```python
from build123d import *

# Parameters (mm, degrees)
EXTRUDE_1_DEPTH                = 500
SKETCH_2_W                     = 500
SKETCH_2_H                     = 30
EXTRUDE_2_DEPTH                = 4.65
CUT_EXTRUDE_1_DEPTH            = 501
CUT_EXTRUDE_2_DEPTH            = 501
SKETCH_5_W                     = 6.7
SKETCH_5_H                     = 0.8
CUT_EXTRUDE_3_DEPTH            = 501
CUT_EXTRUDE_4_DEPTH            = 501
CUT_EXTRUDE_5_DEPTH            = 501
CUT_EXTRUDE_6_DEPTH            = 501
SKETCH_9_W                     = 18.238994336
SKETCH_9_H                     = 8
CUT_EXTRUDE_7_DEPTH            = 501
DRAFT_1_ANGLE                  = 45
DRAFT_2_ANGLE                  = 24.775140569
F_4_2_4_2_DIAMETER_HOLE1_D     = 4.2
F_4_2_4_2_DIAMETER_HOLE1_DEPTH = 500
F_6_0_6_DIAMETER_HOLE1_D       = 6
F_6_0_6_DIAMETER_HOLE1_DEPTH   = 500
CHAMFER_1_SIZE                 = 0.6
CHAMFER_1_SIZE2                = 0.279784595
CHAMFER_2_SIZE                 = 0.6
CHAMFER_3_SIZE                 = 1
CHAMFER_4_SIZE                 = 1.5
FILLET_1_R                     = 3


with BuildPart() as part:
    # 스케치1 → 보스-돌출1 (new body)
    with BuildSketch(Plane(origin=(400, 0, 0), x_dir=(0, 0, -1), z_dir=(1, 0, 0))):
        Polygon((-17.85, 38.2), (-17.85, -0.8), (22.5, -0.8), (22.5, 39.2), (-16.85, 39.2), align=None)
    extrude(amount=-EXTRUDE_1_DEPTH)

    # 스케치2 → 보스-돌출2 (add)
    with BuildSketch(Plane.XY.offset(17.85)):
        with Locations((150, 14.2)):
            Rectangle(SKETCH_2_W, SKETCH_2_H)
    extrude(amount=EXTRUDE_2_DEPTH)

    # 스케치3 → 컷-돌출1 (cut, through all)
    with BuildSketch(Plane.ZY.offset(100)):
        Polygon((22.5, 10.8), (22.5, 15.8), (20.1, 15.8), (20.1, 17.4), (14.9, 17.4), (14.9, 9.2), (20.1, 9.2), (20.1, 10.8), align=None)
    extrude(amount=-CUT_EXTRUDE_1_DEPTH, mode=Mode.SUBTRACT)

    # 스케치4 → 컷-돌출2 (cut, through all)
    with BuildSketch(Plane.ZY.offset(100)):
        Polygon((13.5, -0.8), (18.5, -0.8), (18.5, 1.9), (20.1, 1.9), (20.1, 6.9), (11.9, 6.9), (11.9, 1.9), (13.5, 1.9), align=None)
    extrude(amount=-CUT_EXTRUDE_2_DEPTH, mode=Mode.SUBTRACT)

    # 스케치5 → 컷-돌출3 (cut, through all)
    with BuildSketch(Plane.ZY.offset(100)):
        with Locations((0, -0.4)):
            Rectangle(SKETCH_5_W, SKETCH_5_H)
    extrude(amount=-CUT_EXTRUDE_3_DEPTH, mode=Mode.SUBTRACT)

    # 스케치6 → 컷-돌출4 (cut, through all)
    with BuildSketch(Plane.ZY.offset(100)):
        Polygon((-18.5, -0.8), (-13.5, -0.8), (-13.5, 1.9), (-11.9, 1.9), (-11.9, 6.9), (-20.1, 6.9), (-20.1, 1.9), (-18.5, 1.9), align=None)
    extrude(amount=-CUT_EXTRUDE_4_DEPTH, mode=Mode.SUBTRACT)

    # 스케치7 → 컷-돌출5 (cut, through all)
    with BuildSketch(Plane.ZY.offset(100)):
        Polygon((-22.5, 15.8), (-22.5, 10.8), (-20.1, 10.8), (-20.1, 9.2), (-14.9, 9.2), (-14.9, 17.4), (-20.1, 17.4), (-20.1, 15.8), align=None)
    extrude(amount=-CUT_EXTRUDE_5_DEPTH, mode=Mode.SUBTRACT)

    # 스케치8 → 컷-돌출6 (cut, through all)
    with BuildSketch(Plane.ZY.offset(100)):
        with BuildLine():
            Line((-17.85, 36.705493963), (-17.85, 39.2))
            Line((-17.85, 39.2), (-22.5, 39.2))
            Line((-22.5, 39.2), (-22.5, 29.2))
            Line((-22.5, 29.2), (-17.85, 29.2))
            Line((-17.85, 29.2), (-17.85, 31.694506037))
            ThreePointArc((-17.85, 31.694506037), (-19.2, 34.2), (-17.85, 36.705493963))
        make_face()
    extrude(amount=-CUT_EXTRUDE_6_DEPTH, mode=Mode.SUBTRACT)

    # 스케치9 → 컷-돌출7 (cut, through all)
    with BuildSketch(Plane.ZY.offset(100)):
        with Locations((0, 35.2)):
            Rectangle(SKETCH_9_W, SKETCH_9_H)
    extrude(amount=-CUT_EXTRUDE_7_DEPTH, mode=Mode.SUBTRACT)

    # 구배1
    draft_1_faces = [part.faces().sort_by_distance(p)[0] for p in [
        (150, -0.4, 3.35),
        (150, -0.4, -3.35),
    ]]
    draft(draft_1_faces, Plane(origin=(400, 0, 3.35), x_dir=(0, 0, -1), z_dir=(0, -1, 0)), DRAFT_1_ANGLE)

    # 구배2
    draft_2_faces = [part.faces().sort_by_distance(p)[0] for p in [
        (150, 35.2, 9.119497168),
        (150, 35.2, -9.119497168),
    ]]
    draft(draft_2_faces, Plane(origin=(400, 31.2, -9.119497168), x_dir=(0, 0, 1), z_dir=(0, 1, 0)), DRAFT_2_ANGLE)

    # Ø4.2 (4.2) Diameter Hole1
    with Locations(Plane(origin=(400, 0, 0), x_dir=(0, 0, -1), z_dir=(1, 0, 0))):
        with Locations((-7.5, 5.25), (7.5, 5.25), (0, 26)):
            Hole(F_4_2_4_2_DIAMETER_HOLE1_D / 2, depth=F_4_2_4_2_DIAMETER_HOLE1_DEPTH)

    # Ø6.0 (6) Diameter Hole1
    with Locations(Plane.ZY.offset(100)):
        with Locations((16.290651015, 34.2)):
            Hole(F_6_0_6_DIAMETER_HOLE1_D / 2, depth=F_6_0_6_DIAMETER_HOLE1_DEPTH)

    # 모따기1
    chamfer_1_edges = [part.edges().sort_by_distance(p)[0] for p in [
        (400, 26, -2.1),
        (400, 5.25, -9.6),
        (400, 5.25, 5.4),
    ]]
    chamfer_1_side = [part.faces().sort_by_distance(p)[0] for p in [
        (400, 17.793427641, -0.369480422),
    ]]
    chamfer(chamfer_1_edges, length=CHAMFER_1_SIZE, length2=CHAMFER_1_SIZE2, reference=chamfer_1_side[0])

    # 모따기2
    chamfer_2_edges = [part.edges().sort_by_distance(p)[0] for p in [
        (-100, 26, -2.1),
        (-100, 5.25, -9.6),
        (-100, 5.25, 5.4),
    ]]
    chamfer(chamfer_2_edges, length=CHAMFER_2_SIZE)

    # 모따기3
    chamfer_3_edges = [part.edges().sort_by_distance(p)[0] for p in [
        (150, 39.2, -17.85),
    ]]
    chamfer(chamfer_3_edges, length=CHAMFER_3_SIZE)

    # 모따기4
    chamfer_4_edges = [part.edges().sort_by_distance(p)[0] for p in [
        (150, 29.2, -22.5),
        (150, 29.2, 22.5),
        (150, -0.8, 22.5),
        (150, -0.8, -22.5),
    ]]
    chamfer(chamfer_4_edges, length=CHAMFER_4_SIZE)

    # 필렛1
    fillet_1_edges = [part.edges().sort_by_distance(p)[0] for p in [
        (150, 39.2, -12.811804861),
        (150, 39.2, 12.811804861),
        (150, 31.2, 9.119497168),
        (150, 31.2, -9.119497168),
    ]]
    fillet(fillet_1_edges, radius=FILLET_1_R)


solid = part.part
```
Geometry check sheet. Reference: the model listing, model coordinates, mm. A direction names the side the tool comes from. Round coordinates to 2 decimals unless told otherwise and drop trailing zeros. Return JSON: item names as keys, results as strings. Group by question number.
Q1. Tool access check on faces 1 (the flat face through (146, 31.2, 0)), 2 (the flat face through (147, 22, 22.5)), 3 (the flat face through (146, 6.9, 16)). Record the directions out of +Z, -Z, +X, -X, +Y, -Y that give a thin tool (end or side, any length) a straight path to the whole face; none if there is none.
Q2. Section check A-A, the plane x = 47. Count the separate pieces of the cut face and the enclosed holes in it, plus the area to 3 significant figures.
Q3. Release check for a two-part mould opening along Z. For faces 4 (the flat face through (147, 6, 22.5)), 5 (the flat face through (146, 13, -14.9)), 6 (the flat face through (147, -0.8, 9)), 7 (the flat face through (154, 6, -22.5)) record: released by +Z, released by -Z, zero draft, split by the parting line, or undercut.
Q4. Material ranges on probe 1 along Y at (x, z) = (227, 0); probe 2 along Y at (x, z) = (357, -7); probe 3 along Z at (x, y) = (249, 6), recorded low to high. Write a range as from..to.
Q5. Gauge pin test, flat ends, axial feed: pin 1 (1.9 mm diameter, centred on x = 26, z = 20.5, fed in from +Y); pin 2 (2 mm diameter, centred on x = 38.5, z = -1, fed in from -Y); pin 3 (1.6 mm diameter, centred on x = 63.5, z = -18, fed in from +Y). Record the tip position at first contact, or that the pin passes through.
Numbers:
{
 "1": {"face 1": "+X, -X, +Y", "face 2": "+Z, +X, -X, +Y, -Y", "face 3": "+X, -X"},
 "2": {"separate pieces": "1", "enclosed holes": "3", "area": "1,240 mm^2"},
 "3": {"face 4": "released by +Z", "face 5": "undercut", "face 6": "zero draft", "face 7": "released by -Z"},
 "4": {"probe 1": "0..23.9, 28.1..31.2", "probe 2": "-0.8..3.21, 7.29..31.2", "probe 3": "-22.5..-20.1, -11.9..-9.46, -5.54..5.54, 9.46..11.9, 20.1..22.5"},
 "5": {"pin 1": "y = 29.2", "pin 2": "y = 0", "pin 3": "y = 38.85"}
}
